Design review of the part built by this model. Coordinates are the model's own, in mm. Face numbers are marked on the shaded views. A direction names the side the tool comes from. Coordinates: 2 decimals unless noted, no trailing zeros. Order: outer loops, then holes, each group sorted by start corner. A loop starts at its lowest first (then second) coordinate and runs counter-clockwise, first axis right, second up.
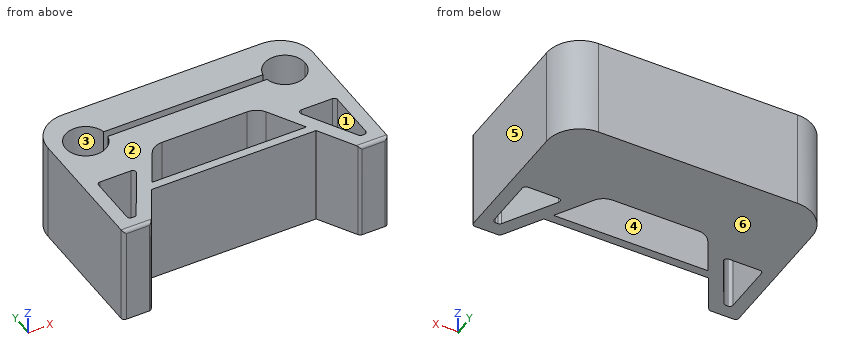
from build123d import *

# Parameters (mm, degrees)
F0_W      = 80
F0_H      = 50
F1_DEPTH  = 30
F3_DEPTH  = 15
F4_R      = 4
F5_DEPTH  = 12
F6_R      = 10
F8_DEPTH  = 30
F9_R      = 5
F11_DEPTH = 32
F12_R     = 1
F13_R     = 1
F14_W     = 7.6178369459
F14_H     = 2.2
F15_DEPTH = 20
F17_DEPTH = 30


with BuildPart() as f1:
    # F0 (on Top) → F1 (new body)
    with BuildSketch(Plane.XY):
        Rectangle(F0_W, F0_H)
    extrude(amount=F1_DEPTH)

    # F2 (on face) → F3 (cut)
    with BuildSketch(Plane.XY.offset(30)):
        with BuildLine():
            ThreePointArc((-26.0503164684, 11.4), (-34.1, 12.5), (-26.0503164684, 13.6))
            Line((-26.0503164684, 13.6), (-24, 13.6))
            ThreePointArc((-24, 13.6), (-36.1, 12.5), (-24, 11.4))
            Line((-24, 11.4), (-26.0503164684, 11.4))
        make_face()
        with BuildLine():
            ThreePointArc((-26.0503164684, 13.6), (-25.9377529322, 13.0551114844), (-25.9, 12.5))
            ThreePointArc((-25.9, 12.5), (-25.9377529322, 11.9448885156), (-26.0503164684, 11.4))
            Line((-26.0503164684, 11.4), (-24, 11.4))
            ThreePointArc((-24, 11.4), (-23.9250514405, 11.9477319491), (-23.9, 12.5))
            ThreePointArc((-23.9, 12.5), (-23.9250514405, 13.0522680509), (-24, 13.6))
            Line((-24, 13.6), (-26.0503164684, 13.6))
        make_face()
        with BuildLine():
            Line((-30, 13.6), (-26.0503164684, 13.6))
            ThreePointArc((-26.0503164684, 13.6), (-34.1, 12.5), (-26.0503164684, 11.4))
            Line((-26.0503164684, 11.4), (-30, 11.4))
            Line((-30, 11.4), (-30, 13.6))
        make_face()
        with BuildLine():
            ThreePointArc((-26.0503164684, 11.4), (-25.9377529322, 11.9448885156), (-25.9, 12.5))
            ThreePointArc((-25.9, 12.5), (-25.9377529322, 13.0551114844), (-26.0503164684, 13.6))
            Line((-26.0503164684, 13.6), (-30, 13.6))
            Line((-30, 13.6), (-30, 11.4))
            Line((-30, 11.4), (-26.0503164684, 11.4))
        make_face()
        with BuildLine():
            Line((-3.8089184729, 13.6), (-24, 13.6))
            ThreePointArc((-24, 13.6), (-23.9250514405, 13.0522680509), (-23.9, 12.5))
            ThreePointArc((-23.9, 12.5), (-23.9250514405, 11.9477319491), (-24, 11.4))
            Line((-24, 11.4), (-3.8089184729, 11.4))
            Line((-3.8089184729, 11.4), (-3.8089184729, 13.6))
        make_face()
        with BuildLine():
            ThreePointArc((36.1, 12.5), (30.5522680509, 18.5749485595), (24, 13.6))
            Line((24, 13.6), (26.0503164684, 13.6))
            ThreePointArc((26.0503164684, 13.6), (30.5551114844, 16.5622470678), (34.1, 12.5))
            ThreePointArc((34.1, 12.5), (30.5551114844, 8.4377529322), (26.0503164684, 11.4))
            Line((26.0503164684, 11.4), (24, 11.4))
            ThreePointArc((24, 11.4), (30.5522680509, 6.4250514405), (36.1, 12.5))
        make_face()
        with BuildLine():
            Line((26.0503164684, 13.6), (24, 13.6))
            ThreePointArc((24, 13.6), (23.9, 12.5), (24, 11.4))
            Line((24, 11.4), (26.0503164684, 11.4))
            ThreePointArc((26.0503164684, 11.4), (25.9, 12.5), (26.0503164684, 13.6))
        make_face()
        with BuildLine():
            Line((30, 13.6), (26.0503164684, 13.6))
            ThreePointArc((26.0503164684, 13.6), (25.9, 12.5), (26.0503164684, 11.4))
            Line((26.0503164684, 11.4), (30, 11.4))
            Line((30, 11.4), (30, 13.6))
        make_face()
        with BuildLine():
            ThreePointArc((34.1, 12.5), (30.5551114844, 16.5622470678), (26.0503164684, 13.6))
            Line((26.0503164684, 13.6), (30, 13.6))
            Line((30, 13.6), (30, 11.4))
            Line((30, 11.4), (26.0503164684, 11.4))
            ThreePointArc((26.0503164684, 11.4), (30.5551114844, 8.4377529322), (34.1, 12.5))
        make_face()
        with BuildLine():
            Line((24, 13.6), (3.8089184729, 13.6))
            Line((3.8089184729, 13.6), (3.8089184729, 11.4))
            Line((3.8089184729, 11.4), (24, 11.4))
            ThreePointArc((24, 11.4), (23.9, 12.5), (24, 13.6))
        make_face()
    extrude(amount=-F3_DEPTH, mode=Mode.SUBTRACT)

    # F4 (on face) → F5 (cut)
    with BuildSketch(Plane.XY.offset(15)):
        with Locations((-30, 12.5)):
            Circle(F4_R)
        with Locations((30, 12.5)):
            Circle(F4_R)
    extrude(amount=-F5_DEPTH, mode=Mode.SUBTRACT)

    # F6
    f6_edges = [f1.edges().sort_by_distance(p)[0] for p in [
        (-40, 25, 15),
        (40, 25, 15),
    ]]
    fillet(f6_edges, radius=F6_R)

    # F7 (on face) → F8 (cut)
    with BuildSketch(Plane.XY.offset(30)):
        Polygon((15.7377014204, 2.2584984545), (-15.7377014204, 2.2584984545), (-31.4754028408, -25), (31.4754028408, -25), align=None)
    extrude(amount=-F8_DEPTH, mode=Mode.SUBTRACT)

    # F9
    f9_edges = [f1.edges().sort_by_distance(p)[0] for p in [
        (15.737701, 2.258498, 15),
        (-15.737701, 2.258498, 15),
    ]]
    fillet(f9_edges, radius=F9_R)

    # F10 (on face) → F11 (cut)
    with BuildSketch(Plane.XY.offset(30)):
        Polygon((-23.9627902868, -4), (-36, -4), (-36, -21), (-33.7840610196, -21), align=None)
        Polygon((36, -4), (23.9627902868, -4), (33.7840610196, -21), (36, -21), align=None)
    extrude(amount=-F11_DEPTH, mode=Mode.SUBTRACT)

    # F12
    f12_edges = [f1.edges().sort_by_distance(p)[0] for p in [
        (-23.96279, -4, 15),
        (-36, -21, 15),
        (-36, -4, 15),
        (-33.784061, -21, 15),
        (23.96279, -4, 15),
        (36, -4, 15),
        (36, -21, 15),
        (33.784061, -21, 15),
    ]]
    fillet(f12_edges, radius=F12_R)

    # F13
    f13_edges = [f1.edges().sort_by_distance(p)[0] for p in [
        (-35.737701, -25, 30),
        (35.737701, -25, 30),
        (-40, -25, 15),
        (-31.475403, -25, 15),
        (31.475403, -25, 15),
        (40, -25, 15),
    ]]
    fillet(f13_edges, radius=F13_R)

    # F14 (on face) → F15 (cut)
    with BuildSketch(Plane.XY.offset(30)):
        with Locations((0, 12.5)):
            Rectangle(F14_W, F14_H)
    extrude(amount=-F15_DEPTH, mode=Mode.SUBTRACT)

    # F16 (on face) → F17 (join)
    with BuildSketch(Plane.XY.offset(30)):
        Polygon((23.3065289789, -10.8510954306), (-23.3065289789, -10.8510954306), (-24.7726006861, -13.390406115), (24.7726006861, -13.390406115), align=None)
    extrude(amount=-F17_DEPTH)


solid = f1.part
1. Add section C-C (y = -2.5). Give the boundary of the cut face in (x, z), and give its area (3 significant figures).
2. Add section D-D (z = 13.75). State how many separate pieces and enclosed holes the cut face has, and give its area (3 significant figures).
3. Add section B-B (y = -12.5). Give the boundary of the cut face in (x, z), and give its area (3 significant figures).
4. To check wall thickness, follow line 1 (Y direction, x = 2, z = 27.75); line 2 (Y direction, x = -0.5, z = 3.75); line 3 (X direction, y = -10, z = 19). State the ranges of each line that lie inside material, in increasing order.
5. Mouldability with a two-part tool opening along X and no side actions: class the marked faces 4, 5 and 6 as pulls with the +X half, pulls with the -X half, needs draft (parallel to the pull), parting line crosses it, or undercut.
6. For the marked faces 1, 2 and 3, list the 3-axis set-ups (+Z, -Z, +X, -X, +Y, -Y) from which the entire face can be reached by the end or side of a thin tool; tool diameter is ignored.
7. Add section A-A (x = 3). Give the boundary of the cut face in (y, z), and give its area (3 significant figures).
8. Insertion check: pin 1 (9 mm diameter, centred on x = -30, y = 12.5, fed in from +Z); pin 2 (1.5 mm diameter, centred on x = 28, z = 9, fed in from -Y); pin 3 (7.5 mm diameter, centred on x = -28, z = 20, fed in from -Y); pin 4 (9 mm diameter, centred on x = 30, y = 12.5, fed in from -Z). Each pin has a flat end and moves straight along its axis. Give the tip position at first contact, or say it passes through.
Solution:
1. outline: (-40, 0) - (-18.49, 0) - (-18.49, 30) - (-40, 30) - close; (18.49, 0) - (40, 0) - (40, 30) - (18.49, 30) - close
1. area: 1,290 mm2
2. separate pieces: 1
2. enclosed holes: 6
2. area: 2,440 mm2
3. outline: (-40, 0) - (-36, 0) - (-36, 30) - (-40, 30) - close; (-28.87, 0) - (28.87, 0) - (28.87, 30) - (-28.87, 30) - close; (36, 0) - (40, 0) - (40, 30) - (36, 30) - close
3. area: 1,970 mm2
4. line 1: y = -13.39 to -10.85, 2.26 to 11.4, 13.6 to 25
4. line 2: y = -13.39 to -10.85, 2.26 to 25
4. line 3: x = -40 to -36, -27.43 to -22.82, 22.82 to 27.43, 36 to 40
5. face 4: undercut
5. face 5: pulls with the +X half
5. face 6: needs draft
6. face 1: +Z, -Z
6. face 2: +Z, +X, -X, +Y, -Y
6. face 3: +Z
7. outline: (-13.39, 0) - (-10.85, 0) - (-10.85, 30) - (-13.39, 30) - close; (2.26, 0) - (25, 0) - (25, 30) - (13.6, 30) - (13.6, 10) - (11.4, 10) - (11.4, 30) - (2.26, 30) - close
7. area: 714 mm2
8. pin 1: stops at z = 15
8. pin 2: stops at y = -20.28
8. pin 3: stops at y = -24.95
8. pin 4: stops at z = 0
